Input: part model. Units: mm. Frame: model coordinates. A direction names the side the tool comes from. Round coordinates to 2 decimals unless told otherwise and drop trailing zeros. Loops run counter-clockwise (first coordinate to the right, second up) from the corner with the lowest first, then second, coordinate; pieces in that order, holes last.
(1) First-contact query: pin 1 Ø1.2 at (x, y) = (0, -0.5) entering from -Z; pin 2 Ø4 at (y, z) = (1, 11) entering from +X; pin 3 Ø1 at (y, z) = (0, 6) entering from -X. Flat tips, straight axial feed; report the tip coordinate or a pass-through.
(2) Cut plane A-A, the plane z = 6.75. Output: boundary loops of the cut face in (x, y), and give its area (3 significant figures).
(3) Line query: line 1 (Z direction, x = 0.5, y = -0.5); line 2 (Z direction, x = -2, y = 4.25); line 3 (Y direction, x = -2.25, z = 8.25). Output: solid intervals per line, ascending.
(4) Draft query along Y for faces 1 (the face through (2.2, 2.2, 0)), 2 (the face through (-2.947, 0.13, 9.614)), 3 (the face through (0, 0, -0.25)). Return one class per face: released by +Y, released by -Y, zero draft, split by the parting line, or undercut.
(5) Access query for faces 4 (the face through (1.014, -1.724, -1.771)), 5 (the face through (0, 0, 20)). Directions: +Z, -Z, +X, -X, +Y, -Y. A direction counts if a zero-diameter tool reaches every point of the face in a straight line with its end or side. Return the directions, or none.
from build123d import *

# Parameters (mm, degrees)
SKIZZE1_R                       = 2.95
AUFSATZ_LINEAR_AUSTRAGEN1_DEPTH = 20
FASE1_SIZE                      = 0.5
SCHNITT_LINEAR_AUSTRAGEN1_DEPTH = 3


with BuildPart() as part:
    # Skizze1 → Aufsatz-Linear austragen1 (new body)
    with BuildSketch(Plane.XY):
        Circle(SKIZZE1_R)
    extrude(amount=AUFSATZ_LINEAR_AUSTRAGEN1_DEPTH)

    # Skizze2 → Rotation1 (revolve)
    with BuildSketch(Plane(origin=(0, 0, 0), x_dir=(0, 0, -1), z_dir=(1, 0, 0)), mode=Mode.PRIVATE) as rotation1_sk:
        with BuildLine():
            Line((3.25, 0), (3.25, 3.1))
            ThreePointArc((3.25, 3.1), (2.122398964, 4.311690857), (0.695193089, 5.15))
            Line((0.695193089, 5.15), (0, 5.15))
            Line((0, 5.15), (0, 0))
            Line((0, 0), (3.25, 0))
        make_face()
    revolve(rotation1_sk.sketch.rotate(Axis((0, 0, 0), (0, 0, -1)), 90), axis=Axis((0, 0, 0), (0, 0, -1)))

    # Fase1
    fase1_edges = [part.edges().sort_by_distance(p)[0] for p in [
        (-2.95, 0, 20),
    ]]
    chamfer(fase1_edges, length=FASE1_SIZE)

    # Skizze3 → Schnitt-Linear austragen1 (cut)
    with BuildSketch(Plane(origin=(0, 0, -3.25), x_dir=(-1, 0, 0), z_dir=(0, 0, -1))):
        Polygon((2, 1.154700538), (0, 2.309401077), (-2, 1.154700538), (-2, -1.154700538), (0, -2.309401077), (2, -1.154700538), align=None)
    extrude(amount=-SCHNITT_LINEAR_AUSTRAGEN1_DEPTH, mode=Mode.SUBTRACT)


solid = part.part
Reported:
1. pin 1: stops at z = -0.25
1. pin 2: stops at x = 2.95
1. pin 3: stops at x = -2.95
2. outline: circle Ø5.9 at (0, 0)
2. area: 27.3 mm2
3. line 1: z = -0.25 to 20
3. line 2: z = -1.58 to 0
3. line 3: y = -1.91 to 1.91
4. face 1: zero draft
4. face 2: split by the parting line
4. face 3: undercut
5. face 4: -Z
5. face 5: +Z, +X, -X, +Y, -Y
